from build123d import *

# Parameters (mm, degrees)
SKETCH1_W           = 13
SKETCH1_H           = 19
BOSS_EXTRUDE1_DEPTH = 22
SKETCH3_R           = 1.5
CUT_EXTRUDE1_DEPTH  = 8
SKETCH4_R           = 1.5
CUT_EXTRUDE2_DEPTH  = 22


with BuildPart() as part:
    # Sketch1 → Boss-Extrude1 (new body)
    with BuildSketch(Plane(origin=(0, 0, 0), x_dir=(1, 0, 0), z_dir=(0, 1, 0))):
        Rectangle(SKETCH1_W, SKETCH1_H)
    extrude(amount=BOSS_EXTRUDE1_DEPTH)

    # Sketch3 → Cut-Extrude1 (cut)
    with BuildSketch(Plane.XY.offset(9.5)):
        with Locations((0, 14)):
            Circle(SKETCH3_R)
        with Locations(Location((0, 8, 0), (0, 0, 180))):
            Circle(SKETCH3_R)
    extrude(amount=-CUT_EXTRUDE1_DEPTH, mode=Mode.SUBTRACT)

    # Sketch4 → Cut-Extrude2 (cut)
    with BuildSketch(Plane(origin=(0, 22, 0), x_dir=(1, 0, 0), z_dir=(0, 1, 0))):
        with Locations(Location((3, 0, 0), (0, 0, 270))):
            Circle(SKETCH4_R)
        with Locations(Location((-3, 0, 0), (0, 0, 270))):
            Circle(SKETCH4_R)
    extrude(amount=-CUT_EXTRUDE2_DEPTH, mode=Mode.SUBTRACT)


solid = part.part
Geometry: final body of the model. Coordinates: model frame, mm. A direction names the side the tool comes from. Give positions to 0.01 mm unless a question says otherwise; leave off trailing zeros. Write each loop counter-clockwise with the first axis right and the second up, starting at its lowest first coordinate (ties: lowest second). Pieces come first, ordered by that corner, then holes.
(1) Cut plane B-B, the plane y = 8. Return loops of the section in (x, z), then the cut area to 3 significant figures.
(2) Cut plane D-D, the plane z = 5.25. Return loops of the section in (x, y), then the cut area to 3 significant figures.
(3) First-contact query: P1, Ø1.8, axis at x = 0, y = 14, coming from the +Z side; P2, Ø2.5, axis at x = 3, z = 0, coming from the +Y side. Flat tips, straight axial feed; report the tip coordinate or a pass-through.
(4) Cut plane A-A, the plane z = 0. Return loops of the section in (x, y).
(5) Mould query, pull axis Z, two halves, no side actions, for faces 3 (the flat face through (0, 11, -9.5)), 4 (the cylindrical face through (-1.513, 11.154, -0.195)), 5 (the flat face through (0, 8, 1.5)). Classes: released by +Z, released by -Z, zero draft, split by the parting line, or undercut.
(6) Ray query, line 1 (Y direction, x = 0, z = 3.5); line 2 (X direction, y = 10.5, z = 0); line 3 (X direction, y = 8, z = 5). Return the intervals inside material, ascending.
(7) Access query for faces 1 (the flat face through (0, 22, 0)), 2 (the flat face through (0, 14, 1.5)). Directions: +Z, -Z, +X, -X, +Y, -Y. A direction counts if a zero-diameter tool reaches every point of the face in a straight line with its end or side. Return the directions, or none.
(8) Cut plane C-C, the plane x = -3.75. Return loops of the section in (y, z).
Values follow:
1. outline: (-6.5, -9.5) - (6.5, -9.5) - (6.5, 9.5) - (1.5, 9.5) - (1.5, 1.5) - (-1.5, 1.5) - (-1.5, 9.5) - (-6.5, 9.5) - close; hole circle Ø3 at (-3, 0); hole circle Ø3 at (3, 0)
1. area: 209 mm2
2. outline: (-6.5, 0) - (6.5, 0) - (6.5, 22) - (-6.5, 22) - close; hole circle Ø3 at (0, 8); hole circle Ø3 at (0, 14)
2. area: 272 mm2
3. P1: stops at z = 1.5
3. P2: passes through
4. outline: (-6.5, 0) - (-4.5, 0) - (-4.5, 22) - (-6.5, 22) - close; (-1.5, 0) - (1.5, 0) - (1.5, 22) - (-1.5, 22) - close; (4.5, 0) - (6.5, 0) - (6.5, 22) - (4.5, 22) - close
5. face 3: released by -Z
5. face 4: undercut
5. face 5: released by +Z
6. line 1: y = 0 to 6.5, 9.5 to 12.5, 15.5 to 22
6. line 2: x = -6.5 to -4.5, -1.5 to 1.5, 4.5 to 6.5
6. line 3: x = -6.5 to -1.5, 1.5 to 6.5
7. face 1: +Z, -Z, +X, -X, +Y
7. face 2: +Z
8. outline: (0, -9.5) - (22, -9.5) - (22, -1.3) - (0, -1.3) - close; (0, 1.3) - (22, 1.3) - (22, 9.5) - (0, 9.5) - close
